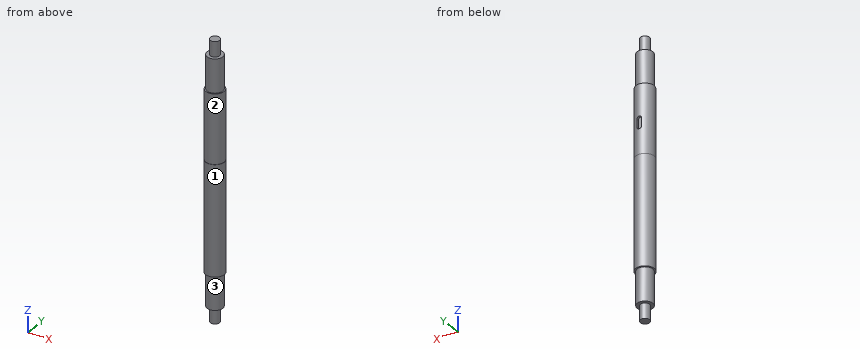
from build123d import *

# Parameters (mm, degrees)
SKETCH1_R           = 9.525
BOSS_EXTRUDE1_DEPTH = 139.7
CUT_EXTRUDE1_REACH  = 232.645
SKETCH3_R           = 9.525
SKETCH3_R_2         = 7.9375
CUT_EXTRUDE2_REACH  = 266.503
SKETCH4_R           = 7.9375
SKETCH4_R_2         = 4.7625
SKETCH5_R           = 9.525
SKETCH5_R_2         = 9.2075
CUT_EXTRUDE3_DEPTH  = 69.85
CUT_EXTRUDE4_DEPTH  = 2.38125


with BuildPart() as part:
    # Sketch1 → Boss-Extrude1 (new, symmetric)
    with BuildSketch(Plane.XY):
        Circle(SKETCH1_R)
    extrude(amount=BOSS_EXTRUDE1_DEPTH, both=True)

    # Sketch3 → Cut-Extrude1 (cut, up to next)
    with BuildSketch(Plane.XY.offset(90.551), mode=Mode.PRIVATE) as cut_extrude1_sk1:
        Circle(SKETCH3_R)
        Circle(SKETCH3_R_2, mode=Mode.SUBTRACT)
    cut_extrude1_tool1 = extrude(cut_extrude1_sk1.sketch, amount=CUT_EXTRUDE1_REACH, mode=Mode.PRIVATE) & part.part
    cut_extrude1 = cut_extrude1_tool1.solids().sort_by_distance((-9.255592, 0, 90.551))[0]
    add(cut_extrude1, mode=Mode.SUBTRACT)

    # Mirror1: Cut-Extrude1 across plane
    add(cut_extrude1.mirror(Plane.XY), mode=Mode.SUBTRACT)

    # Sketch4 → Cut-Extrude2 (cut, up to next)
    with BuildSketch(Plane.XY.offset(124.46), mode=Mode.PRIVATE) as cut_extrude2_sk1:
        Circle(SKETCH4_R)
        with Locations(Location((0, 0, 0), (0, 0, 180))):
            Circle(SKETCH4_R_2, mode=Mode.SUBTRACT)
    cut_extrude2_tool1 = extrude(cut_extrude2_sk1.sketch, amount=CUT_EXTRUDE2_REACH, mode=Mode.PRIVATE) & part.part
    cut_extrude2 = cut_extrude2_tool1.solids().sort_by_distance((-7.712994, 0, 124.46))[0]
    add(cut_extrude2, mode=Mode.SUBTRACT)

    # Mirror2: Cut-Extrude2 across plane
    add(cut_extrude2.mirror(Plane.XY), mode=Mode.SUBTRACT)

    # Sketch5 → Cut-Extrude3 (cut)
    with BuildSketch(Plane.XY.offset(90.551)):
        Circle(SKETCH5_R)
        Circle(SKETCH5_R_2, mode=Mode.SUBTRACT)
    extrude(amount=-CUT_EXTRUDE3_DEPTH, mode=Mode.SUBTRACT)

    # Sketch6 → Cut-Extrude4 (cut)
    with BuildSketch(Plane(origin=(0, 9.2075, 0), x_dir=(1, 0, 0), z_dir=(0, 1, 0))):
        with BuildLine():
            Line((2.38125, -56.41975), (2.38125, -48.48225))
            ThreePointArc((2.38125, -48.48225), (0, -46.101), (-2.38125, -48.48225))
            Line((-2.38125, -48.48225), (-2.38125, -56.41975))
            ThreePointArc((-2.38125, -56.41975), (0, -58.801), (2.38125, -56.41975))
        make_face()
    extrude(amount=-CUT_EXTRUDE4_DEPTH, mode=Mode.SUBTRACT)


solid = part.part
Model file for the job. Use its own axes, mm. Face numbers are marked on the shaded views. A direction names the side the tool comes from. Give positions to 0.01 mm unless a question says otherwise; leave off trailing zeros. Order: outer loops, then holes, each group sorted by start corner. A loop starts at its lowest first (then second) coordinate and runs counter-clockwise, first axis right, second up. Notation, with made-up numbers: M -40,21 L 6,21 A35 ccw 6,53 Z; hole C -4.75,77 d6. An arc over 180 degrees is marked long. Put each result on its own line as item: value. Start each with the question number.
(1) Drill centre lines: L1, parallel to Y at x = 0.75, z = -77; L2, parallel to X at y = -2.5, z = -34.5; L3, parallel to Z at x = -4.5, y = 5.25. Where is each one in solid material? Low to high. Write a range as [from, to].
(2) Pin check, flat tips, straight feed: pin 1 Ø0.6 at (y, z) = (8, 53) entering from +X; pin 2 Ø1 at (y, z) = (-2, -50) entering from -X; pin 3 Ø6 at (x, z) = (-7, -36) entering from -Y. Stop position of each tip, or through.
(3) Band-saw the part on D-D on z = 16.5. Give the cut face in (x, y) (3 decimals).
(4) Tool access for the marked faces 1, 2 and 3: list every direction of +Z, -Z, +X, -X, +Y, -Y with a clear straight run to the whole face (end or side of a thin tool).
(5) Band-saw the part on C-C on z = 87. Give the cut face in (x, y) (1 decimal).
Results below:
1. L1: y = [-9.5, 9.5]
1. L2: x = [-9.19, 9.19]
1. L3: z = [-124.46, 124.46]
2. pin 1: stops at x = 5.05
2. pin 2: stops at x = -9.41
2. pin 3: stops at y = -8.64
3. outline: C 0,0 d19.05
4. face 1: +Z, -Z
4. face 2: +Z
4. face 3: -Z
5. outline: C 0,0 d18.4
